Source: three-view drawing plus pictorial views. Frame: mm from the lowest corner of the part. A direction names the side the tool comes from. Give positions to 0.01 mm unless a question says otherwise; leave off trailing zeros. Loops run counter-clockwise (first coordinate to the right, second up) from the corner with the lowest first, then second, coordinate; pieces in that order, holes last. Notation, with made-up numbers: (-34.5, 85) - (0.5, 85) arc R17 cw to (0.5, 117) - close; hole circle Ø9 at (77.25, 78.25). An arc over 180 degrees is marked (long way). Answer as a JSON object with one key per item and string values. Group by question number.
(1) Section query D-D (z = 10). Return loops of the section in (x, y), plus the area to 3 significant figures.
(2) Section query A-A (y = 17). Return loops of the section in (x, z), plus the area to 4 significant figures.
(3) Access query for the marked faces 1 and 2. Directions: +Z, -Z, +X, -X, +Y, -Y. A direction counts if a zero-diameter tool reaches every point of the face in a straight line with its end or side. Return the directions, or none.
(4) Section query B-B (z = 72). Return loops of the section in (x, y).
(5) Material intervals for L1, parallel to X at y = 3.4, z = 72; L2, parallel to Y at x = 1, z = 30; L3, parallel to Z at x = 42, y = 2.45, sorted ascending.
(6) Pin query (flat end, axial travel): P1, Ø6, axis at y = 40, z = 50, coming from the -X side; P2, Ø3, axis at y = 44, z = 14.5, coming from the +X side; P3, Ø13.5, axis at x = 16.5, z = 36, coming from the +Y side. Return the tip coordinate at first contact, or that it passes through.
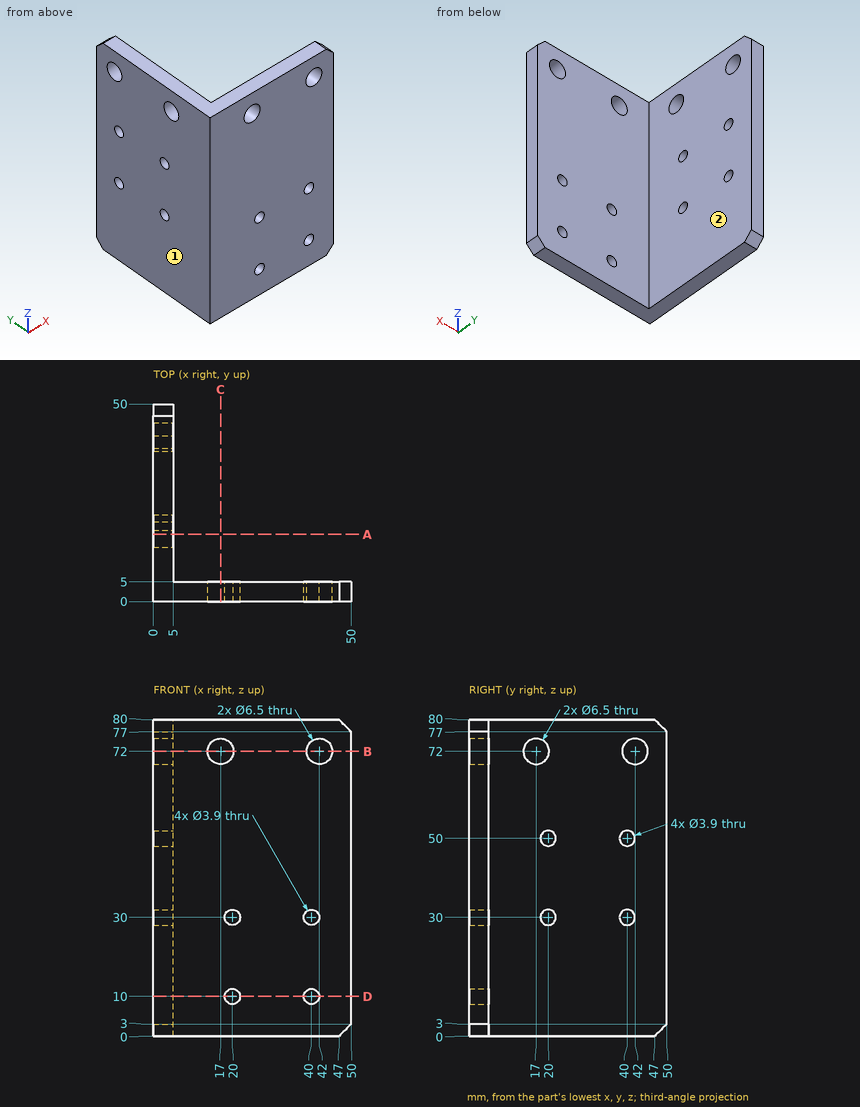
Recorded:
{
 "1": {"outline": "(0, 0) - (18.05, 0) - (18.05, 5) - (5, 5) - (5, 50) - (0, 50) - close; (21.95, 0) - (38.05, 0) - (38.05, 5) - (21.95, 5) - close; (41.95, 0) - (50, 0) - (50, 5) - (41.95, 5) - close", "area": "436 mm^2"},
 "2": {"outline": "(0, 0) - (5, 0) - (5, 68.75) - (0, 68.75) - close; (0, 75.25) - (5, 75.25) - (5, 80) - (0, 80) - close", "area": "367.5 mm^2"},
 "3": {"face 1": "+Z, -Z, -X, +Y, -Y", "face 2": "+Z, -Z, +X, +Y"},
 "4": {"outline": "(0, 0) - (13.75, 0) - (13.75, 5) - (5, 5) - (5, 13.75) - (0, 13.75) - close; (0, 20.25) - (5, 20.25) - (5, 38.75) - (0, 38.75) - close; (0, 45.25) - (5, 45.25) - (5, 50) - (0, 50) - close; (20.25, 0) - (38.75, 0) - (38.75, 5) - (20.25, 5) - close; (45.25, 0) - (50, 0) - (50, 5) - (45.25, 5) - close"},
 "5": {"L1": "x = 0 to 13.75, 20.25 to 38.75, 45.25 to 50", "L2": "y = 0 to 18.05, 21.95 to 38.05, 41.95 to 50", "L3": "z = 0 to 68.75, 75.25 to 80"},
 "6": {"P1": "stops at x = 0", "P2": "stops at x = 5", "P3": "stops at y = 5"}
}
